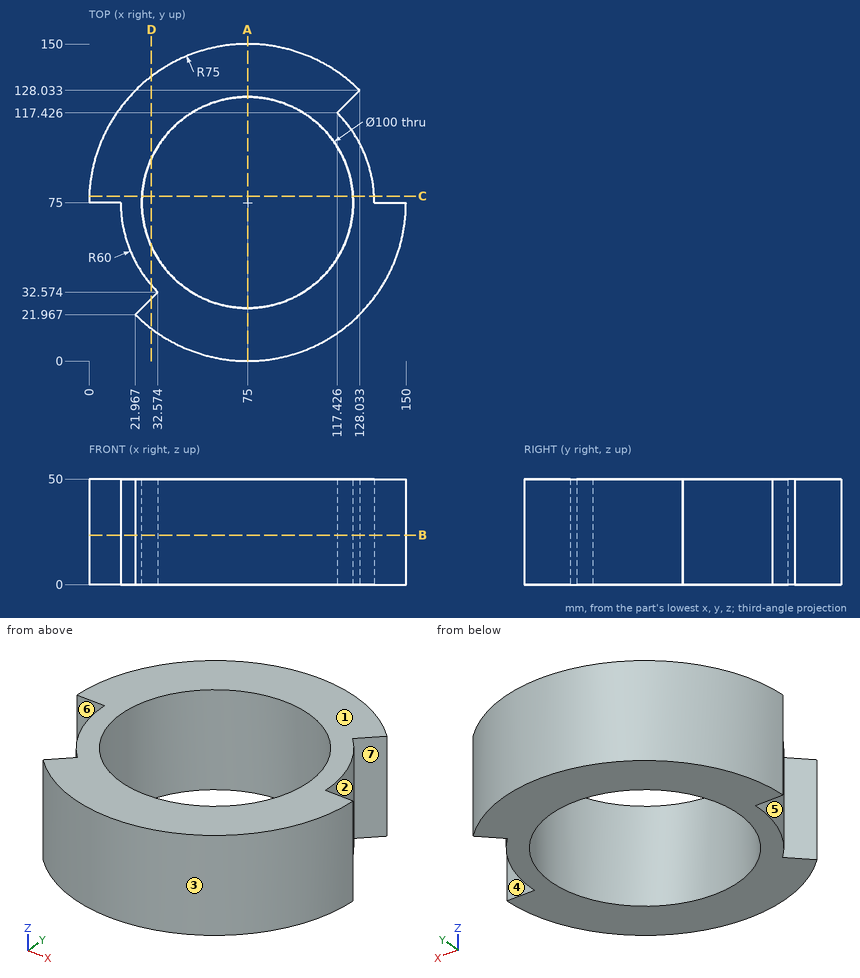
Geometry check sheet. Reference: drawing and pictorial views, mm from the part's lowest x, y, z. A direction names the side the tool comes from. Give positions to 0.01 mm unless a question says otherwise; leave off trailing zeros. Order: outer loops, then holes, each group sorted by start corner. A loop starts at its lowest first (then second) coordinate and runs counter-clockwise, first axis right, second up. Notation, with made-up numbers: M 27.25,87.5 L 37.25,87.5 A32 ccw 37.25,125.5 Z; hole C -16.5,21.25 d7. An arc over 180 degrees is marked long. Answer in a Markdown table with one row per item. Add a question column.
Item 1: Section check B-B, the plane z = 23.5. Enter the section's corners in (x, y).
Item 2: Gauge pin test, flat ends, axial feed: pin 1 (3 mm diameter, centred on y = 119, z = 15, fed in from +X); pin 2 (5 mm diameter, centred on y = 97, z = 43.5, fed in from +X); pin 3 (8 mm diameter, centred on y = 79.5, z = 15, fed in from +X). Record the tip position at first contact, or that the pin passes through.
Item 3: Section check D-D, the plane x = 29.5. Enter the section's corners in (y, z).
Item 4: Section check A-A, the plane x = 75. Enter the section's corners in (y, z), and give its area (3 significant figures).
Item 5: Tool access check on the marked faces 4, 5, 6 and 7. Record the directions out of +Z, -Z, +X, -X, +Y, -Y that give a thin tool (end or side, any length) a straight path to the whole face; none if there is none.
Item 6: Scan lines: probe 1 along X at (y, z) = (77, 16); probe 2 along Y at (x, z) = (75, 30); probe 3 along Y at (x, z) = (85, 26). Record each from-to range of solid material in increasing order. Write a range as from..to.
Item 7: Mould release check, pull along Y, two halves, no side actions. Record for the marked faces 1, 2 and 3: released by +Y, released by -Y, zero draft, split by the parting line, or undercut.
Item 8: Section check C-C, the plane y = 78. Enter the section's corners in (x, z) (1 decimal).
Filled sheet:
| question | item | result |
|---|---|---|
| 1 | outline | M 0,75 L 15,75 A60 ccw 32.57,32.57 L 21.97,21.97 A75 ccw 150,75 L 135,75 A60 ccw 117.43,117.43 L 128.03,128.03 A75 ccw Z; hole C 75,75 d100 |
| 2 | pin 1 | stops at x = 120.5 |
| 2 | pin 2 | stops at x = 131.74 |
| 2 | pin 3 | stops at x = 135 |
| 3 | outline | M 15.38,0 L 29.5,0 L 29.5,50 L 15.38,50 Z; M 35.89,0 L 54.27,0 L 54.27,50 L 35.89,50 Z; M 95.73,0 L 134.62,0 L 134.62,50 L 95.73,50 Z |
| 4 | outline | M 0,0 L 25,0 L 25,50 L 0,50 Z; M 125,0 L 150,0 L 150,50 L 125,50 Z |
| 4 | area | 2,500 mm^2 |
| 5 | face 4 | +Z, -Z, +X, +Y |
| 5 | face 5 | +Z, -Z, -X |
| 5 | face 6 | +Z, -Z, -X, -Y |
| 5 | face 7 | +Z, -Z, +X |
| 6 | probe 1 | x = 0.03..25.04, 124.96..134.97 |
| 6 | probe 2 | y = 0..25, 125..150 |
| 6 | probe 3 | y = 0.67..26.01, 123.99..149.33 |
| 7 | face 1 | zero draft |
| 7 | face 2 | undercut |
| 7 | face 3 | released by -Y |
| 8 | outline | M 0.1,0 L 25.1,0 L 25.1,50 L 0.1,50 Z; M 124.9,0 L 134.9,0 L 134.9,50 L 124.9,50 Z |
